Could you check a few things on this model? Use its own coordinates, in mm. Face numbers are marked on the shaded views. Coordinates: 2 decimals unless noted, no trailing zeros. Order: outer loops, then holes, each group sorted by start corner. A loop starts at its lowest first (then second) coordinate and runs counter-clockwise, first axis right, second up. Notation, with made-up numbers: (75, 56.25) -> (104, 56.25) arc R19 cw to (104, 90.25) -> close; hole circle Ø2 at (25.5, 40). An arc over 180 degrees is marked (long way). Use a Markdown table: item, result. Add a question column.
1) If we section it at B-B (x = 0): Write out the boundary of the cut face in (y, z).
2) If I drill on L1, parallel to Z at x = 0, y = 2.55; L2, parallel to X at y = 1.2, z = 0; L3, parallel to X at y = 2.2, z = 7 (3 decimals), over which ranges is the centre line in solid material (lowest first)? Write a range as [from, to].
3) Thinking about a two-plate mould opening in X: for the marked faces 1, 2 and 3, which applies, +X half, -X half, draft (parallel to the pull), parting line (faces both ways), or undercut?
4) If we section it at D-D (z = -15.25): Write out the boundary of the cut face in (x, y).
5) Will these pins go through, and if not, where does the flat tip stop? pin 1 Ø1 at (x, y) = (5.5, 0.5) entering from +Z; pin 2 Ø2 at (y, z) = (1, 6) entering from +X.
6) If we section it at A-A (z = 0): Write out the boundary of the cut face in (x, y), plus the area to 3 significant figures.
7) If we section it at C-C (y = 2.95): Give the number of separate pieces and of enclosed holes in the cut face, plus the area to 3 significant figures.
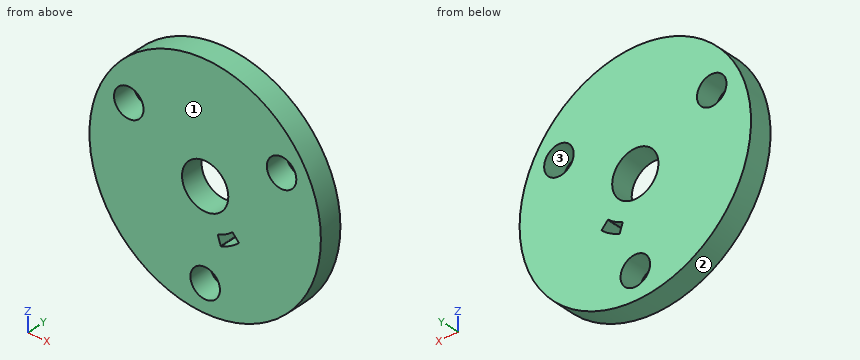
```python
from build123d import *

# Parameters (mm, degrees)
SKETCH1_R           = 20
SKETCH1_R_2         = 4
BOSS_EXTRUDE1_DEPTH = 4
SKETCH2_R           = 2.55
CUT_EXTRUDE2_DEPTH  = 5
CIRPATTERN1_COUNT   = 3
CUT_EXTRUDE3_DEPTH  = 5
FILLET1_R           = 0.1


with BuildPart() as part:
    # Sketch1 → Boss-Extrude1 (new body)
    with BuildSketch(Plane(origin=(0, 0, 0), x_dir=(1, 0, 0), z_dir=(0, 1, 0))):
        Circle(SKETCH1_R)
        Circle(SKETCH1_R_2, mode=Mode.SUBTRACT)
    extrude(amount=BOSS_EXTRUDE1_DEPTH)

    # Sketch2 → Cut-Extrude2 (cut, through all)
    with BuildSketch(Plane(origin=(0, 4, 0), x_dir=(1, 0, 0), z_dir=(0, 1, 0))):
        with Locations((0, 15.25)):
            Circle(SKETCH2_R)
    cut_extrude2 = extrude(amount=-CUT_EXTRUDE2_DEPTH, mode=Mode.SUBTRACT)

    # CirPattern1: Cut-Extrude2 ×3 about axis
    cirpattern1_axis = Axis((0, 0, 0), (0, 1, 0))
    for i in range(1, CIRPATTERN1_COUNT):
        add(cut_extrude2.rotate(cirpattern1_axis, i * 360 / CIRPATTERN1_COUNT), mode=Mode.SUBTRACT)

    # Sketch3 → Cut-Extrude3 (cut, through all)
    with BuildSketch(Plane(origin=(0, 4, 0), x_dir=(1, 0, 0), z_dir=(0, 1, 0))):
        with BuildLine():
            Line((2.703898701, 8.321744518), (2.17856981, 6.70494844))
            ThreePointArc((2.17856981, 6.70494844), (3.525, 6.105479097), (4.717370775, 5.23917102))
            Line((4.717370775, 5.23917102), (5.854892806, 6.502517223))
            ThreePointArc((5.854892806, 6.502517223), (4.375, 7.577722283), (2.703898701, 8.321744518))
        make_face()
    extrude(amount=-CUT_EXTRUDE3_DEPTH, mode=Mode.SUBTRACT)

    # Fillet1
    fillet1_edges = [part.edges().sort_by_distance(p)[0] for p in [
        (2.703898701, 2, -8.321744518),
        (5.854892806, 2, -6.502517223),
        (4.717370775, 2, -5.23917102),
        (2.17856981, 2, -6.70494844),
    ]]
    fillet(fillet1_edges, radius=FILLET1_R)


solid = part.part
```
Answer sheet:
| question | item | result |
|---|---|---|
| 1 | outline | (0, -20) -> (4, -20) -> (4, -17.8) -> (0, -17.8) -> close; (0, -12.7) -> (4, -12.7) -> (4, -4) -> (0, -4) -> close; (0, 4) -> (4, 4) -> (4, 20) -> (0, 20) -> close |
| 2 | L1 | [-20, -17.8], [-12.7, -4], [4, 20] |
| 2 | L2 | [-20, -4], [4, 20] |
| 2 | L3 | [-18.735, -15.679], [-10.735, 10.735], [15.679, 18.735] |
| 3 | face 1 | draft |
| 3 | face 2 | parting line |
| 3 | face 3 | undercut |
| 4 | outline | (-12.94, 0) -> (-2.55, 0) -> (-2.55, 4) -> (-12.94, 4) -> close; (2.55, 0) -> (12.94, 0) -> (12.94, 4) -> (2.55, 4) -> close |
| 5 | pin 1 | z = 19.36 |
| 5 | pin 2 | x = 19.36 |
| 6 | outline | (-20, 0) -> (-4, 0) -> (-4, 4) -> (-20, 4) -> close; (4, 0) -> (20, 0) -> (20, 4) -> (4, 4) -> close |
| 6 | area | 128 mm2 |
| 7 | separate pieces | 1 |
| 7 | enclosed holes | 5 |
| 7 | area | 1,140 mm2 |
